```python
from build123d import *

# Parameters (mm, degrees)
BOSS_EXTRUDE5_DEPTH = 10
CUT_EXTRUDE6_DEPTH  = 5
FILLET4_R           = 1
MIRROR25_DEPTH      = 10
MIRROR25_2_DEPTH    = 5
SKETCH20_W          = 13.27
SKETCH20_H          = 33.288518674
CUT_EXTRUDE7_DEPTH  = 10


# Read off the part's stored shape, not the designer's step: Mirror25
with BuildPart() as part:
    # Sketch15 → Boss-Extrude5 (new body)
    with BuildSketch(Plane(origin=(0, 0, 0), x_dir=(1, 0, 0), z_dir=(0, 1, 0))):
        Polygon((24.3, 76.900659127), (-6.625, 76.900659127), (-6.625, -4.5), (24.3, -4.5), (24.3, 44.900659127), (21.675, 44.900659127), (21.675, 47.400659127), (21.675, 72.400659127), (21.675, 74.900659127), (24.3, 74.900659127), align=None)
        Polygon((-2.625, 25), (-2.625, 0), (-2.625, -2.5), (0, -2.5), (2.625, -2.5), (2.625, 0), (2.625, 25), (2.625, 27.5), (0, 27.5), (-2.625, 27.5), align=None, mode=Mode.SUBTRACT)
    extrude(amount=BOSS_EXTRUDE5_DEPTH)

    # Sketch18 → Cut-Extrude6 (cut)
    with BuildSketch(Plane(origin=(0, 10, 0), x_dir=(1, 0, 0), z_dir=(0, 1, 0))):
        Polygon((21.675, 51.3980649), (-4.44053483, 51.3980649), (-4.44053483, 20.8980649), (24.3, 20.8980649), (24.3, 51.3980649), align=None)
    extrude(amount=-CUT_EXTRUDE6_DEPTH, mode=Mode.SUBTRACT)

    # Fillet4
    fillet4_edges = [part.edges().sort_by_distance(p)[0] for p in [
        (21.675, 5, -74.900659127),
        (-2.625, 5, 2.5),
        (2.625, 5, 2.5),
        (2.625, 2.5, -27.5),
        (-2.625, 2.5, -27.5),
        (21.675, 2.5, -44.900659127),
    ]]
    fillet(fillet4_edges, radius=FILLET4_R)

    # Mirror25 outline → Mirror25 (add)
    with BuildSketch(Plane(origin=(0, 0, 0), x_dir=(1, 0, 0), z_dir=(0, 1, 0))):
        with BuildLine():
            Line((45.975, 20.8980649), (24.3, 20.8980649))
            Line((24.3, 20.8980649), (24.3, -4.5))
            Line((24.3, -4.5), (55.225, -4.5))
            Line((55.225, -4.5), (55.225, 76.900659127))
            Line((55.225, 76.900659127), (24.3, 76.900659127))
            Line((24.3, 76.900659127), (24.3, 74.900659127))
            Line((24.3, 74.900659127), (25.925, 74.900659127))
            ThreePointArc((25.925, 74.900659127), (26.632106781, 74.607765908), (26.925, 73.900659127))
            Line((26.925, 73.900659127), (26.925, 51.3980649))
            Line((26.925, 51.3980649), (53.04053483, 51.3980649))
            Line((53.04053483, 51.3980649), (53.04053483, 20.8980649))
            Line((53.04053483, 20.8980649), (51.225, 20.8980649))
            Line((51.225, 20.8980649), (51.225, -1.5))
            ThreePointArc((51.225, -1.5), (50.932106781, -2.207106781), (50.225, -2.5))
            Line((50.225, -2.5), (46.975, -2.5))
            ThreePointArc((46.975, -2.5), (46.267893219, -2.207106781), (45.975, -1.5))
            Line((45.975, -1.5), (45.975, 20.8980649))
        make_face()
    extrude(amount=MIRROR25_DEPTH)

    # Mirror25 2 outline → Mirror25 2 (add)
    with BuildSketch(Plane(origin=(0, 0, 0), x_dir=(1, 0, 0), z_dir=(0, 1, 0))):
        with BuildLine():
            Line((25.925, 44.900659127), (24.3, 44.900659127))
            Line((24.3, 44.900659127), (24.3, 20.8980649))
            Line((24.3, 20.8980649), (45.975, 20.8980649))
            Line((45.975, 20.8980649), (45.975, 26.5))
            ThreePointArc((45.975, 26.5), (46.267893219, 27.207106781), (46.975, 27.5))
            Line((46.975, 27.5), (50.225, 27.5))
            ThreePointArc((50.225, 27.5), (50.932106781, 27.207106781), (51.225, 26.5))
            Line((51.225, 26.5), (51.225, 20.8980649))
            Line((51.225, 20.8980649), (53.04053483, 20.8980649))
            Line((53.04053483, 20.8980649), (53.04053483, 51.3980649))
            Line((53.04053483, 51.3980649), (26.925, 51.3980649))
            Line((26.925, 51.3980649), (26.925, 45.900659127))
            ThreePointArc((26.925, 45.900659127), (26.632106781, 45.193552346), (25.925, 44.900659127))
        make_face()
    extrude(amount=MIRROR25_2_DEPTH)

    # Sketch20 → Cut-Extrude7 (cut)
    with BuildSketch(Plane(origin=(0, 10, 0), x_dir=(1, 0, 0), z_dir=(0, 1, 0))):
        with Locations((13.258799085, 2.964933045)):
            Rectangle(SKETCH20_W, SKETCH20_H)
        Polygon((-6.625, 76.900659127), (14.49053483, 76.900659127), (14.49053483, 89.151488298), (21.675, 89.151488298), (26.925, 89.151488298), (29.3, 89.151488298), (29.3, 51.3980649), (26.925, 51.3980649), (26.925, 61.088659891), (21.675, 61.088659891), (21.675, 51.3980649), (-4.44053483, 51.3980649), (-4.44053483, 42.900659127), (-6.625, 42.900659127), (-6.625, 56.002594228), align=None)
    extrude(amount=-CUT_EXTRUDE7_DEPTH, mode=Mode.SUBTRACT)


solid = part.part
```
Build history of the part. All positions in model axes, mm. A direction names the side the tool comes from. Round coordinates to 2 decimals unless told otherwise and drop trailing zeros. Write each loop counter-clockwise with the first axis right and the second up, starting at its lowest first coordinate (ties: lowest second). Pieces come first, ordered by that corner, then holes. Notation, with made-up numbers: (81.25, 12.5) - (137.25, 12.5) arc R22 ccw to (137.25, 43.5) - close; hole circle Ø3 at (-29, 2.25). An arc over 180 degrees is marked (long way). Write each question's results on one line, items separated by ' | '. Start each with the question number.
Item 1: Saw through at A-A (z = -12). Write the cut outline in (x, y) (3 decimals).
Item 2: Saw through at D-D (x = 39.5). Write the cut outline in (y, z), and give its area (3 significant figures).
Item 3: Wall check: L1, parallel to X at y = 4, z = -23 (3 decimals); L2, parallel to X at y = 9, z = -13 (3 decimals); L3, parallel to X at y = 9.5, z = -32 (3 decimals). Give the ranges that are in metal, low to high. Write a range as [from, to].
Item 4: Mould opens along X. For faces 1 (the face through (2.625, 5, -13)), 2 (the face through (41, 7, -51.398)) say: pulls with the +X half, pulls with the -X half, needs draft (parallel to the pull), parting line crosses it, or undercut.
Item 5: Which spindle directions (+Z, -Z, +X, -X, +Y, -Y) get a long thin tool onto all of the face, cutting with end or side? Do faces 3 (the face through (53.041, 7, -36)), 4 (the face through (45.975, 5, -12)), 5 (the face through (21.675, 2, -49)), 6 (the face through (-4, 8, -20.898)), 7 (the face through (28, 3, -51.398)). Say none if no direction does.
Item 6: Saw through at B-B (z = -24.5). Write the cut outline in (x, y) (3 decimals), and give its area (3 significant figures).
Item 7: Drop flat-ended pins along their axis: P1, Ø1, axis at x = 0.5, y = 6, coming from the -Z side; P2, Ø1.5, axis at x = 20.5, y = 4, coming from the -Z side; P3, Ø2.5, axis at x = 24, y = 3.5, coming from the -Z side. Give the stop position or say it passes through.
Item 8: Saw through at C-C (y = 1). State how many separate pieces and enclosed holes the cut face has, and give its area (3 significant figures).
Results are:
1) outline: (-6.625, 0) - (-2.625, 0) - (-2.625, 10) - (-6.625, 10) - close; (2.625, 0) - (6.624, 0) - (6.624, 10) - (2.625, 10) - close; (19.894, 0) - (45.975, 0) - (45.975, 10) - (19.894, 10) - close; (51.225, 0) - (55.225, 0) - (55.225, 10) - (51.225, 10) - close
2) outline: (0, -76.9) - (10, -76.9) - (10, -51.4) - (5, -51.4) - (5, -20.9) - (10, -20.9) - (10, 4.5) - (0, 4.5) - close | area: 662 mm²
3) L1: x = [-6.625, -2.625], [2.625, 45.975], [51.225, 55.225] | L2: x = [-6.625, -2.625], [2.625, 6.624], [19.894, 45.975], [51.225, 55.225] | L3: x = [-6.625, -4.441], [53.041, 55.225]
4) face 1: undercut | face 2: needs draft
5) face 3: +Y | face 4: +Y, -Y | face 5: -Z, +Y, -Y | face 6: -Z, +Y | face 7: -Z, -X, +Y, -Y
6) outline: (-6.625, 0) - (-2.625, 0) - (-2.625, 5) - (-4.441, 5) - (-4.441, 10) - (-6.625, 10) - close; (2.625, 0) - (45.975, 0) - (45.975, 5) - (2.625, 5) - close; (51.225, 0) - (55.225, 0) - (55.225, 10) - (53.041, 10) - (53.041, 5) - (51.225, 5) - close | area: 279 mm²
7) P1: stops at z = 2.5 | P2: stops at z = -51.4 | P3: stops at z = -44.9
8) separate pieces: 1 | enclosed holes: 2 | area: 3,430 mm²
